Design review of the part built by this model. Coordinates are the model's own, in mm. Face numbers are marked on the shaded views. A direction names the side the tool comes from. Round coordinates to 2 decimals unless told otherwise and drop trailing zeros. Loops run counter-clockwise (first coordinate to the right, second up) from the corner with the lowest first, then second, coordinate; pieces in that order, holes last. Notation, with made-up numbers: (-18, -32.5) - (17, -32.5) arc R12 ccw to (17, -15.5) - close; hole circle Ø6 at (56, 82). An arc over 180 degrees is marked (long way). Answer as CSV lines item,"result". Start each with the question number.
(1) Consider section D-D (x = 0). Give the boundary of the cut face in (y, z).
(2) For the marked faces 4 and 5, list the 3-axis set-ups (+Z, -Z, +X, -X, +Y, -Y) from which the entire face can be reached by the end or side of a thin tool; tool diameter is ignored.
(3) Mouldability with a two-part tool opening along Z and no side actions: class the marked faces 1, 2 and 3 as released by +Z, released by -Z, zero draft, split by the parting line, or undercut.
(4) Consider section C-C (x = -14). Give the boundary of the cut face in (y, z).
(5) Consider section A-A (y = 0). Give the boundary of the cut face in (x, z), and give its area (3 significant figures).
(6) Wall thickness on L1, parallel to Z at x = -14, y = 0; L2, parallel to X at y = -6.5, z = 9.5; L3, parallel to X at y = 13, z = 7.5: over which ranges is each line inside the solid? List them lowest first.
(7) Consider section B-B (z = 9.5). Give the boundary of the cut face in (x, y), and give its area (3 significant figures).
(8) For P1, Ø5, axis at x = 5, y = -1, coming from the -Z side; P2, Ø8, axis at x = 11.5, y = -4.5, coming from the +Z side, all flat-tipped, find the tip position at first contact; note any pin that passes through.
Autodesk Inventor part; units mm, degrees
ref_plane "YZ Plane" through (0, 0, 0) normal (1, 0, 0) x (0, 1, 0)
ref_plane "XZ Plane" through (0, 0, 0) normal (0, 1, 0) x (-1, 0, 0)
ref_plane "XY Plane" through (0, 0, 0) normal (0, 0, 1) x (1, 0, 0)
sketch "Sketch2" plane through (0, 0, 0) normal (0, 0, 1) x (1, 0, 0)
  line L0 (-25, 16) -> (25, 16)
  line L1 (25, 16) -> (25, -16)
  line L2 (25, -16) -> (-25, -16)
  line L3 (-25, -16) -> (-25, 16)
  line L4 (-25, 16) -> (25, -16) construction
  line L5 (25, 16) -> (-25, -16) construction
  point P0 (0, 0)
  dimension "d4" = 32
  dimension "d5" = 50
extrude "Extrusion1" add sketch "Sketch2" along normal blind 26
sketch "Sketch3" plane through (0, 0, 26) normal (0, 0, 1) x (1, 0, 0)
  circle A0 centre (0, 0) radius 7
  dimension "d8" = 14
extrude "Extrusion2" add sketch "Sketch3" along normal blind 3
sketch "Sketch4" plane through (0, 0, 29) normal (0, 0, 1) x (1, 0, 0)
  circle A0 centre (0, 0) radius 4.95
  dimension "d11" = 9.9
extrude "Extrusion3" add sketch "Sketch4" along normal blind 9
sketch "Sketch6" plane through (-25, 16, 0) normal (0, 1, 0) x (1, 0, 0)
  line L0 (11, -9.5) -> (0, -9.5) construction
  line L1 (0, 0) -> (0, -26)
  line L2 (39, -9.5) -> (50, -9.5) construction
  line L3 (50, 0) -> (50, -26)
  line L4 (50, 0) -> (0, 0)
  point P0 (25, 0)
  point P1 (44.5, -9.5)
  dimension "d29" = 28
  dimension "d30" = 9.5
hole "Hole3" at (-14, 16, 9.5) at (14, 16, 9.5) direction (0, -1, 0) diameter 8.2 end through all
properties part number "13042026-03"
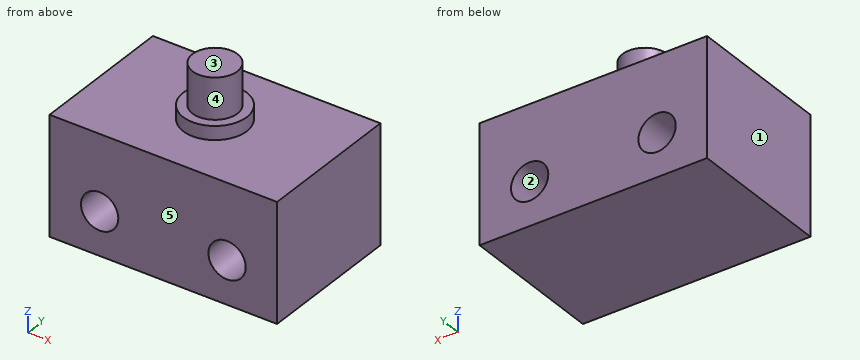
Determined:
1,outline,"(-16, 0) - (16, 0) - (16, 26) - (7, 26) - (7, 29) - (4.95, 29) - (4.95, 38) - (-4.95, 38) - (-4.95, 29) - (-7, 29) - (-7, 26) - (-16, 26) - close"
2,face 4,"+Z"
2,face 5,"+Z, -Z, +X, -X, -Y"
3,face 1,"zero draft"
3,face 2,"undercut"
3,face 3,"released by +Z"
4,outline,"(-16, 0) - (16, 0) - (16, 5.4) - (-16, 5.4) - close; (-16, 13.6) - (16, 13.6) - (16, 26) - (-16, 26) - close"
5,outline,"(-25, 0) - (25, 0) - (25, 26) - (7, 26) - (7, 29) - (4.95, 29) - (4.95, 38) - (-4.95, 38) - (-4.95, 29) - (-7, 29) - (-7, 26) - (-25, 26) - close; hole circle Ø8.2 at (-14, 9.5); hole circle Ø8.2 at (14, 9.5)"
5,area,"1,330 mm^2"
6,L1,"z = 0 to 5.4, 13.6 to 26"
6,L2,"x = -25 to -18.1, -9.9 to 9.9, 18.1 to 25"
6,L3,"x = -25 to -17.58, -10.42 to 10.42, 17.58 to 25"
7,outline,"(-25, -16) - (-18.1, -16) - (-18.1, 16) - (-25, 16) - close; (-9.9, -16) - (9.9, -16) - (9.9, 16) - (-9.9, 16) - close; (18.1, -16) - (25, -16) - (25, 16) - (18.1, 16) - close"
7,area,"1,080 mm^2"
8,P1,"stops at z = 0"
8,P2,"stops at z = 26"
